Read the model definition and answer for the solid it produces. Units are mm, in the model's axes. Face numbers are marked on the shaded views. Coordinates: 2 decimals unless noted, no trailing zeros. Order: outer loops, then holes, each group sorted by start corner. A loop starts at its lowest first (then second) coordinate and runs counter-clockwise, first axis right, second up. Notation, with made-up numbers: M 78,44.5 L 135,44.5 A28 ccw 135,78.5 Z; hole C 42,-4.75 d7. An arc over 180 degrees is marked long. One line per question, with ' | ' between items. Start each with the question number.
1) Consider probe 1 along Z at (x, y) = (-40.66, -5.5); probe 2 along X at (y, z) = (-2.75, 40.66); probe 3 along X at (y, z) = (6.55, 0). Determine where each line is inside the solid, lowest interval first.
2) The mould has two halves that part along X. Classify the marked faces 1 and 2: +X half, -X half, draft (parallel to the pull), parting line (faces both ways), or undercut.
3) Find section D-D, the plane x = 83.5. Write down the section's boundary in (y, z), plus the area to 3 significant figures.
4) Find section B-B, the plane x = 0. Write down the section's boundary in (y, z).
5) Find section C-C, the plane z = -27.5. Write down the section's boundary in (x, y), plus the area to 3 significant figures.
6) Find section A-A, the plane z = 107. Write down the section's boundary in (x, y), plus the area to 4 significant figures.
7) Given P1, Ø1.5, axis at x = 26.5, z = -24, coming from the +Y side; P2, Ø5.5, axis at x = -23.5, y = -6, coming from the -Z side; P3, Ø2, axis at y = 1, z = -37, coming from the +X side, each flat-ended and moving along its own axis, determine where each tip first touches the part or whether it passes through.
from build123d import *

# Parameters (mm, degrees)
SKETCH1_R            = 125
BOSS_EXTRUDE1_DEPTH  = 3
SKETCH2_R            = 122.5
SKETCH2_R_2          = 112.5
BOSS_EXTRUDE2_DEPTH  = 6
SKETCH3_W            = 94.5
SKETCH3_H            = 94.5
BOSS_EXTRUDE3_DEPTH  = 8
M4_CLEARANCE_HOLE1_D = 4.5
FILLET1_R            = 3
SKETCH8_W            = 21
SKETCH8_H            = 21
BOSS_EXTRUDE4_DEPTH  = 5
FILLET2_R            = 6
FILLET3_R            = 23


with BuildPart() as part:
    # Sketch1 → Boss-Extrude1 (new body)
    with BuildSketch(Plane(origin=(0, 0, 0), x_dir=(1, 0, 0), z_dir=(0, 1, 0))):
        with Locations(Location((0, 0, 0), (0, 0, 270))):
            Circle(SKETCH1_R)
    extrude(amount=BOSS_EXTRUDE1_DEPTH)

    # Sketch2 → Boss-Extrude2 (add)
    with BuildSketch(Plane(origin=(0, 3, 0), x_dir=(1, 0, 0), z_dir=(0, 1, 0))):
        with Locations(Location((0, 0, 0), (0, 0, 270))):
            Circle(SKETCH2_R)
        with Locations(Location((0, 0, 0), (0, 0, 270))):
            Circle(SKETCH2_R_2, mode=Mode.SUBTRACT)
    extrude(amount=BOSS_EXTRUDE2_DEPTH)

    # Sketch3 → Boss-Extrude3 (add)
    with BuildSketch(Plane.XZ):
        Rectangle(SKETCH3_W, SKETCH3_H)
    extrude(amount=BOSS_EXTRUDE3_DEPTH)

    # M4 Clearance Hole1 (through all)
    with Locations(Plane(origin=(0, -8, 0), x_dir=(-1, 0, 0), z_dir=(0, -1, 0))):
        with Locations((40.66, 40.66), (40.66, -40.66), (-40.66, -40.66), (-40.66, 40.66)):
            Hole(M4_CLEARANCE_HOLE1_D / 2)

    # Fillet1
    fillet1_edges = [part.edges().sort_by_distance(p)[0] for p in [
        (0, 0, -47.25),
        (-47.25, 0, 0),
        (0, 0, 47.25),
        (47.25, 0, 0),
    ]]
    fillet(fillet1_edges, radius=FILLET1_R)

    # Sketch8 → Boss-Extrude4 (add)
    with BuildSketch(Plane(origin=(0, 0, 0), x_dir=(-1, 0, 0), z_dir=(0, -1, 0))):
        with Locations((75.1, 0)):
            Rectangle(SKETCH8_W, SKETCH8_H)
    extrude(amount=BOSS_EXTRUDE4_DEPTH)

    # Fillet2
    # the kernel refuses this fillet: 6 mm, written as the material it adds along each edge
    with BuildSketch(Plane(origin=(-64.6, 0, 10.5), x_dir=(1, 0, 0), z_dir=(0, 0, -1)), Plane(origin=(-85.6, 0, 10.5), x_dir=(0, 0, 1), z_dir=(1, 0, 0)), Plane(origin=(-85.6, 0, -10.5), x_dir=(-1, 0, 0), z_dir=(0, 0, 1)), Plane(origin=(-64.6, 0, -10.5), x_dir=(0, 0, -1), z_dir=(-1, 0, 0))) as fillet2_piece_1:
        with BuildLine():
            CenterArc((5.916079783, 6), FILLET2_R, 189.594068227, 80.405931773)
            Line((0, 5), (-0.118321596, 4.98))
            ThreePointArc((-0.118321596, 4.98), (-0.12, 2.5), (-0.12, 0))
            Line((-0.12, 0), (0, -0.12))
            Line((0, -0.12), (5.916079783, -0.12))
            Line((5.916079783, -0.12), (5.916079783, 0))
        make_face()
    extrude(amount=21)
    with BuildSketch(Plane(origin=(-85.6, 0, 10.5), x_dir=(0, 0, 1), z_dir=(1, 0, 0))) as fillet2_piece_2a_section:
        with BuildLine():
            CenterArc((5.916079783, 6), FILLET2_R, 189.594068227, 80.405931773)
            Line((0, 5), (-0.118321596, 4.98))
            ThreePointArc((-0.118321596, 4.98), (-0.12, 2.5), (-0.12, 0))
            Line((-0.12, 0), (0, -0.12))
            Line((0, -0.12), (5.916079783, -0.12))
            Line((5.916079783, -0.12), (5.916079783, 0))
        make_face()
    fillet2_piece_2a = extrude(amount=35.790199458, mode=Mode.PRIVATE)
    fillet2_piece_2a = split(fillet2_piece_2a, bisect_by=Plane(origin=(-64.6, -1.233917871, 11.87196406), z_dir=(1, 0, 0)), keep=Keep.TOP, mode=Mode.PRIVATE)
    with BuildSketch(Plane(origin=(-64.6, 0, 25.290199458), x_dir=(1, 0, 0), z_dir=(0, 0, -1))) as fillet2_piece_2b_section:
        with BuildLine():
            CenterArc((5.916079783, 6), FILLET2_R, 189.594068227, 80.405931773)
            Line((0, 5), (-0.118321596, 4.98))
            ThreePointArc((-0.118321596, 4.98), (-0.12, 2.5), (-0.12, 0))
            Line((-0.12, 0), (0, -0.12))
            Line((0, -0.12), (5.916079783, -0.12))
            Line((5.916079783, -0.12), (5.916079783, 0))
        make_face()
    fillet2_piece_2b = extrude(amount=35.790199458, mode=Mode.PRIVATE)
    fillet2_piece_2b = split(fillet2_piece_2b, bisect_by=Plane(origin=(-63.22803594, -1.233917871, 10.5), z_dir=(0, 0, 1)), keep=Keep.TOP, mode=Mode.PRIVATE)
    fillet2_piece_2 = fillet2_piece_2a & fillet2_piece_2b
    add(fillet2_piece_2)
    with BuildSketch(Plane(origin=(-64.6, 0, 10.5), x_dir=(1, 0, 0), z_dir=(0, 0, -1))) as fillet2_piece_3a_section:
        with BuildLine():
            CenterArc((5.916079783, 6), FILLET2_R, 189.594068227, 80.405931773)
            Line((0, 5), (-0.118321596, 4.98))
            ThreePointArc((-0.118321596, 4.98), (-0.12, 2.5), (-0.12, 0))
            Line((-0.12, 0), (0, -0.12))
            Line((0, -0.12), (5.916079783, -0.12))
            Line((5.916079783, -0.12), (5.916079783, 0))
        make_face()
    fillet2_piece_3a = extrude(amount=35.790199458, mode=Mode.PRIVATE)
    fillet2_piece_3a = split(fillet2_piece_3a, bisect_by=Plane(origin=(-63.22803594, -1.233917871, -10.5), z_dir=(0, 0, -1)), keep=Keep.TOP, mode=Mode.PRIVATE)
    with BuildSketch(Plane(origin=(-49.809800542, 0, -10.5), x_dir=(0, 0, -1), z_dir=(-1, 0, 0))) as fillet2_piece_3b_section:
        with BuildLine():
            CenterArc((5.916079783, 6), FILLET2_R, 189.594068227, 80.405931773)
            Line((0, 5), (-0.118321596, 4.98))
            ThreePointArc((-0.118321596, 4.98), (-0.12, 2.5), (-0.12, 0))
            Line((-0.12, 0), (0, -0.12))
            Line((0, -0.12), (5.916079783, -0.12))
            Line((5.916079783, -0.12), (5.916079783, 0))
        make_face()
    fillet2_piece_3b = extrude(amount=35.790199458, mode=Mode.PRIVATE)
    fillet2_piece_3b = split(fillet2_piece_3b, bisect_by=Plane(origin=(-64.6, -1.233917871, -11.87196406), z_dir=(1, 0, 0)), keep=Keep.TOP, mode=Mode.PRIVATE)
    fillet2_piece_3 = fillet2_piece_3a & fillet2_piece_3b
    add(fillet2_piece_3)
    with BuildSketch(Plane(origin=(-100.390199458, 0, 10.5), x_dir=(0, 0, 1), z_dir=(1, 0, 0))) as fillet2_piece_4a_section:
        with BuildLine():
            CenterArc((5.916079783, 6), FILLET2_R, 189.594068227, 80.405931773)
            Line((0, 5), (-0.118321596, 4.98))
            ThreePointArc((-0.118321596, 4.98), (-0.12, 2.5), (-0.12, 0))
            Line((-0.12, 0), (0, -0.12))
            Line((0, -0.12), (5.916079783, -0.12))
            Line((5.916079783, -0.12), (5.916079783, 0))
        make_face()
    fillet2_piece_4a = extrude(amount=35.790199458, mode=Mode.PRIVATE)
    fillet2_piece_4a = split(fillet2_piece_4a, bisect_by=Plane(origin=(-85.6, -1.233917871, 11.87196406), z_dir=(-1, 0, 0)), keep=Keep.TOP, mode=Mode.PRIVATE)
    with BuildSketch(Plane(origin=(-85.6, 0, -10.5), x_dir=(-1, 0, 0), z_dir=(0, 0, 1))) as fillet2_piece_4b_section:
        with BuildLine():
            CenterArc((5.916079783, 6), FILLET2_R, 189.594068227, 80.405931773)
            Line((0, 5), (-0.118321596, 4.98))
            ThreePointArc((-0.118321596, 4.98), (-0.12, 2.5), (-0.12, 0))
            Line((-0.12, 0), (0, -0.12))
            Line((0, -0.12), (5.916079783, -0.12))
            Line((5.916079783, -0.12), (5.916079783, 0))
        make_face()
    fillet2_piece_4b = extrude(amount=35.790199458, mode=Mode.PRIVATE)
    fillet2_piece_4b = split(fillet2_piece_4b, bisect_by=Plane(origin=(-86.97196406, -1.233917871, 10.5), z_dir=(0, 0, 1)), keep=Keep.TOP, mode=Mode.PRIVATE)
    fillet2_piece_4 = fillet2_piece_4a & fillet2_piece_4b
    add(fillet2_piece_4)
    with BuildSketch(Plane(origin=(-64.6, 0, -10.5), x_dir=(0, 0, -1), z_dir=(-1, 0, 0))) as fillet2_piece_5a_section:
        with BuildLine():
            CenterArc((5.916079783, 6), FILLET2_R, 189.594068227, 80.405931773)
            Line((0, 5), (-0.118321596, 4.98))
            ThreePointArc((-0.118321596, 4.98), (-0.12, 2.5), (-0.12, 0))
            Line((-0.12, 0), (0, -0.12))
            Line((0, -0.12), (5.916079783, -0.12))
            Line((5.916079783, -0.12), (5.916079783, 0))
        make_face()
    fillet2_piece_5a = extrude(amount=35.790199458, mode=Mode.PRIVATE)
    fillet2_piece_5a = split(fillet2_piece_5a, bisect_by=Plane(origin=(-85.6, -1.233917871, -11.87196406), z_dir=(-1, 0, 0)), keep=Keep.TOP, mode=Mode.PRIVATE)
    with BuildSketch(Plane(origin=(-85.6, 0, -25.290199458), x_dir=(-1, 0, 0), z_dir=(0, 0, 1))) as fillet2_piece_5b_section:
        with BuildLine():
            CenterArc((5.916079783, 6), FILLET2_R, 189.594068227, 80.405931773)
            Line((0, 5), (-0.118321596, 4.98))
            ThreePointArc((-0.118321596, 4.98), (-0.12, 2.5), (-0.12, 0))
            Line((-0.12, 0), (0, -0.12))
            Line((0, -0.12), (5.916079783, -0.12))
            Line((5.916079783, -0.12), (5.916079783, 0))
        make_face()
    fillet2_piece_5b = extrude(amount=35.790199458, mode=Mode.PRIVATE)
    fillet2_piece_5b = split(fillet2_piece_5b, bisect_by=Plane(origin=(-86.97196406, -1.233917871, -10.5), z_dir=(0, 0, -1)), keep=Keep.TOP, mode=Mode.PRIVATE)
    fillet2_piece_5 = fillet2_piece_5a & fillet2_piece_5b
    add(fillet2_piece_5)

    # Fillet3
    fillet3_edges = [part.edges().sort_by_distance(p)[0] for p in [
        (-85.6, -5, 0),
        (-75.1, -5, -10.5),
        (-64.6, -5, 0),
        (-75.1, -5, 10.5),
    ]]
    fillet(fillet3_edges, radius=FILLET3_R)


solid = part.part
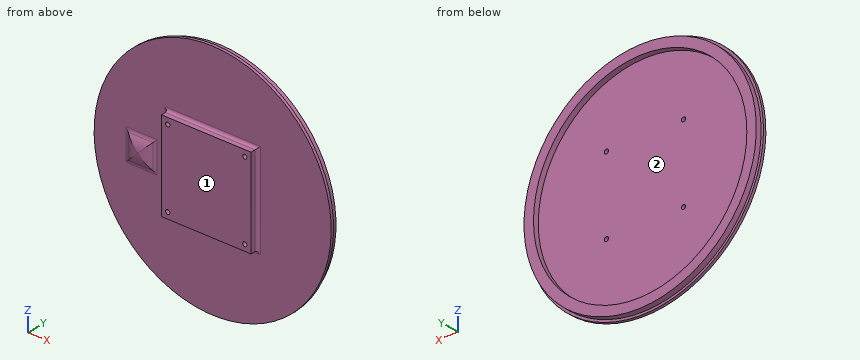
Report:
1) probe 1: z = -47.25 to -42.91, -38.41 to 38.41, 42.91 to 47.25 | probe 2: x = -47.26 to -42.91, -38.41 to 38.41, 42.91 to 47.26 | probe 3: x = -122.5 to -112.5, 112.5 to 122.5
2) face 1: draft | face 2: undercut
3) outline: M 0,-93.02 L 3,-93.02 L 3,-89.63 L 9,-89.63 L 9,-75.39 L 3,-75.39 L 3,75.39 L 9,75.39 L 9,89.63 L 3,89.63 L 3,93.02 L 0,93.02 Z | area: 729 mm^2
4) outline: M -8,-47.25 L -3,-47.25 A3 cw 0,-50.25 L 0,-125 L 3,-125 L 3,-122.5 L 9,-122.5 L 9,-112.5 L 3,-112.5 L 3,112.5 L 9,112.5 L 9,122.5 L 3,122.5 L 3,125 L 0,125 L 0,50.25 A3 cw -3,47.25 L -8,47.25 Z
5) outline: M -121.94,0 L -50.25,0 A3 cw -47.25,-3 L -47.25,-8 L 47.25,-8 L 47.25,-3 A3 cw 50.25,0 L 121.94,0 L 121.94,3 L 119.37,3 L 119.37,9 L 109.09,9 L 109.09,3 L -109.09,3 L -109.09,9 L -119.37,9 L -119.37,3 L -121.94,3 Z | area: 1,610 mm^2
6) outline: M -64.62,0 L 64.62,0 L 64.62,3 L 59.64,3 L 59.64,9 L 34.75,9 L 34.75,3 L -34.75,3 L -34.75,9 L -59.64,9 L -59.64,3 L -64.62,3 Z | area: 686.5 mm^2
7) P1: stops at y = 3 | P2: stops at z = -47.25 | P3: stops at x = 119.7
